The drawing under review shows one solid part. Ordinate dimensions are in mm from its lowest x, y, z. Coordinates: 2 decimals unless noted, no trailing zeros. Write each loop counter-clockwise with the first axis right and the second up, starting at its lowest first coordinate (ties: lowest second). Pieces come first, ordered by that corner, then holes. Notation, with made-up numbers: (-4.5, -23) - (9.5, -23) arc R27 cw to (9.5, -7) - close; hole circle Ø10 at (39, 42.5). An arc over 180 degrees is marked (long way). Put each result on its own line as item: value. Start each with the question number.
Item 1: Mouldability with a two-part tool opening along X and no side actions: class the marked faces 1, 2 and 3 as pulls with the +X half, pulls with the -X half, needs draft (parallel to the pull), parting line crosses it, or undercut.
Item 2: Consider section D-D on x = 6.25. Give the boundary of the cut face in (y, z).
Item 3: Consider section B-B on z = 22. Give the boundary of the cut face in (x, y).
Item 4: Consider section A-A on y = 9. Give the boundary of the cut face in (x, z), then the cut area to 3 significant figures.
Item 5: To check wall thickness, follow L1, parallel to X at y = 11.5, z = 10.75; L2, parallel to X at y = 18, z = 8; L3, parallel to Y at x = 11, z = 6.25. State the ranges of each line that lie inside material, in increasing order. Write a range as [from, to].
Item 6: Consider section C-C on x = 9. Give the boundary of the cut face in (y, z).
Item 7: For pin 1 (1.5 mm diameter, centred on y = 8, z = 19.5, fed in from +X); pin 2 (2 mm diameter, centred on x = 3, z = 20.5, fed in from -Y); pin 3 (8 mm diameter, centred on x = 23, z = 14.5, fed in from +Y); pin 4 (6 mm diameter, centred on y = 17, z = 18.5, fed in from -X), all flat-tipped, find the tip position at first contact; note any pin that passes through.
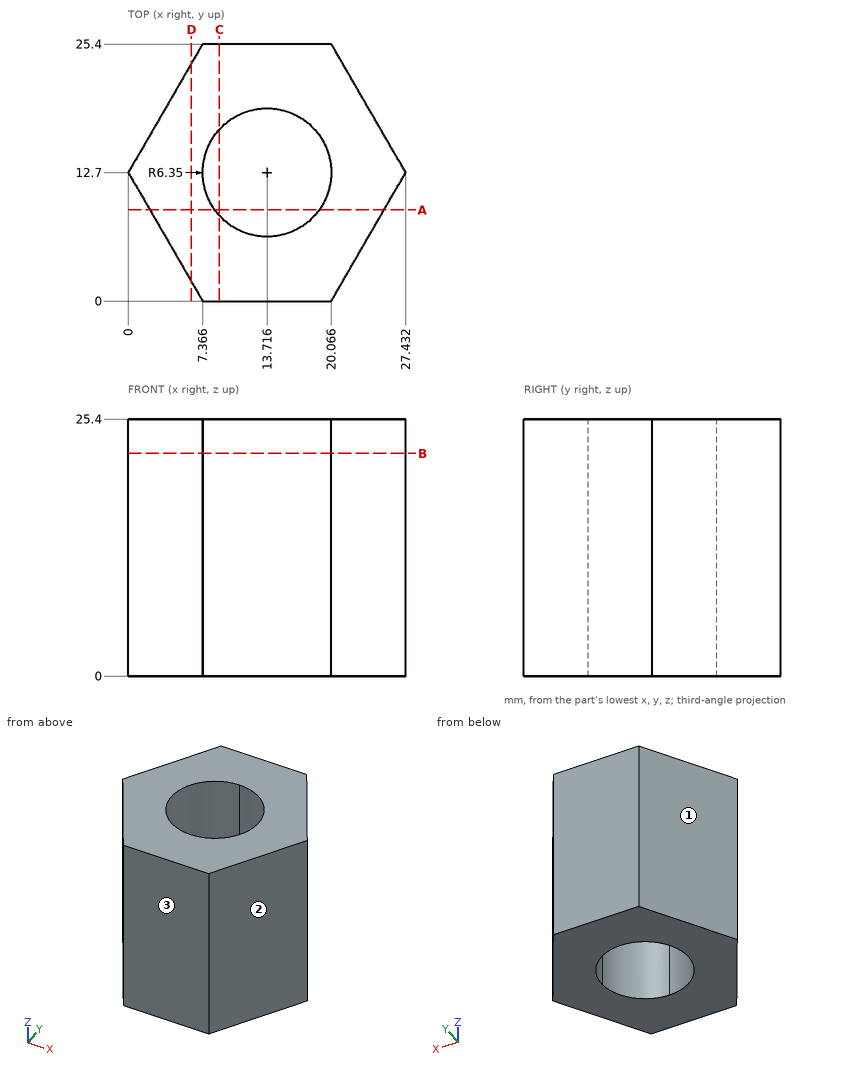
Report:
1. face 1: pulls with the -X half
1. face 2: pulls with the +X half
1. face 3: needs draft
2. outline: (1.92, 0) - (23.48, 0) - (23.48, 25.4) - (1.92, 25.4) - close
3. outline: (0, 12.7) - (7.37, 0) - (20.07, 0) - (27.43, 12.7) - (20.07, 25.4) - (7.37, 25.4) - close; hole circle Ø12.7 at (13.72, 12.7)
4. outline: (2.15, 0) - (8.56, 0) - (8.56, 25.4) - (2.15, 25.4) - close; (18.88, 0) - (25.29, 0) - (25.29, 25.4) - (18.88, 25.4) - close
4. area: 326 mm²
5. L1: [0.7, 7.48], [19.95, 26.74]
5. L2: [3.07, 10.22], [17.21, 24.36]
5. L3: [0, 6.96], [18.44, 25.4]
6. outline: (0, 0) - (8.45, 0) - (8.45, 25.4) - (0, 25.4) - close; (16.95, 0) - (25.4, 0) - (25.4, 25.4) - (16.95, 25.4) - close
7. pin 1: x = 25.14
7. pin 2: y = 5.8
7. pin 3: y = 25.4
7. pin 4: x = 0.75
